from build123d import *

# Parameters (mm, degrees)
SKETCH1_W                    = 60
SKETCH1_H                    = 65
BASE_FLANGE1_DEPTH           = 0.5
CUT_EXTRUDE1_DEPTH           = 45.232341109
EDGE_FLANGE1_STRIP_W         = 2.2
EDGE_FLANGE1_STRIP_H         = 0.5
EDGE_FLANGE1_STRIP_CUT_DEPTH = 65
EDGE_FLANGE1_DEPTH           = 65
EXTRUDE_THIN1_START          = 38.85
EXTRUDE_THIN1_DEPTH          = 38.85
SKETCH87_W                   = 65
SKETCH87_H                   = 10
CUT_EXTRUDE2_DEPTH           = 30


# Sheet-metal steps are written as plain solids
with BuildPart() as part:
    # Sketch1 → Base-Flange1 (new body)
    with BuildSketch(Plane(origin=(0, 0, 0), x_dir=(1, 0, 0), z_dir=(0, 1, 0))):
        Rectangle(SKETCH1_W, SKETCH1_H)
    extrude(amount=-BASE_FLANGE1_DEPTH)

    # Sketch7 → Cut-Extrude1 (cut, through all)
    with BuildSketch(Plane.XZ.offset(0.5)):
        with BuildLine():
            Line((2, 32.5), (-30, 32.5))
            Line((-30, 32.5), (-30, -32.5))
            Line((-30, -32.5), (2, -32.5))
            ThreePointArc((2, -32.5), (-29.169489574, 0), (2, 32.5))
        make_face()
    extrude(amount=-CUT_EXTRUDE1_DEPTH, mode=Mode.SUBTRACT)

    # Edge-Flange1 strip (across the edge) → Edge-Flange1 strip cut (cut)
    with BuildSketch(Plane(origin=(30, -0.5, -32.5), x_dir=(-1, 0, 0), z_dir=(0, 0, 1))):
        with Locations((-0.5, -0.25)):
            Rectangle(EDGE_FLANGE1_STRIP_W, EDGE_FLANGE1_STRIP_H)
    extrude(amount=EDGE_FLANGE1_STRIP_CUT_DEPTH, mode=Mode.SUBTRACT)

    # Edge-Flange1 section (across the edge) → Edge-Flange1 (add)
    with BuildSketch(Plane(origin=(30, -0.5, -32.5), x_dir=(-1, 0, 0), z_dir=(0, 0, 1))):
        with BuildLine():
            Line((0, 0.1), (0, 38.85))
            Line((0, 38.85), (0.5, 38.85))
            Line((0.5, 38.85), (0.5, 0.1))
            ThreePointArc((0.5, 0.1), (0.529289322, 0.029289322), (0.6, 0))
            Line((0.6, 0), (0.6, -0.5))
            ThreePointArc((0.6, -0.5), (0.175735931, -0.324264069), (0, 0.1))
        make_face()
    extrude(amount=EDGE_FLANGE1_DEPTH)

    # Sketch84 → Extrude-Thin1 (add)
    with BuildSketch(Plane.XZ.offset(0.5).offset(EXTRUDE_THIN1_START)):
        with BuildLine():
            Line((29.5, 32.5), (2, 32.5))
            ThreePointArc((2, 32.5), (-29.169489574, 0), (2, -32.5))
            Line((2, -32.5), (29.5, -32.5))
            Line((29.5, -32.5), (29.5, -32))
            Line((29.5, -32), (2.010489053, -32))
            ThreePointArc((2.010489053, -32), (-28.669489574, 0), (2.010489053, 32))
            Line((2.010489053, 32), (29.5, 32))
            Line((29.5, 32), (29.5, 32.5))
        make_face()
    extrude(amount=-EXTRUDE_THIN1_DEPTH)

    # Sketch87 → Cut-Extrude2 (cut)
    with BuildSketch(Plane.ZY.offset(29.169489574)):
        with Locations((0, -21.5)):
            Rectangle(SKETCH87_W, SKETCH87_H)
    extrude(amount=-CUT_EXTRUDE2_DEPTH, mode=Mode.SUBTRACT)


solid = part.part
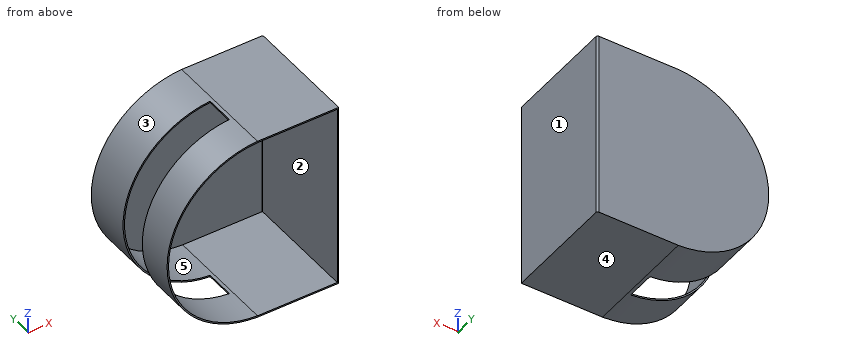
Work out the finished part from the listing and answer in its coordinate system (mm). Face numbers are marked on the shaded views. A direction names the side the tool comes from. Coordinates: 2 decimals unless noted, no trailing zeros. Write each loop counter-clockwise with the first axis right and the second up, starting at its lowest first coordinate (ties: lowest second). Pieces come first, ordered by that corner, then holes. Notation, with made-up numbers: M 26.5,31 L 79.5,31 A27 ccw 79.5,66 Z; hole C -26,-1.5 d3. An arc over 180 degrees is marked long. Use one line per item in the form item = value. Start each with the question number.
1. The part is cut by section D-D (y = -19). Give the vertices of the cut face in (x, z).
2. The part is cut by section B-B (y = -10.5). Give the vertices of the cut face in (x, z).
3. Each of these flat-tipped pins is pushed along its axis until it touches: P1, Ø8, axis at x = 17.5, z = 13, coming from the -Y side; P2, Ø1, axis at y = -30.5, z = -3.5, coming from the -X side; P3, Ø0.6, axis at y = -22, z = -32.5, coming from the -X side. Where does it stop, or does it pass through?
4. The part is cut by section C-C (x = -6.5). Give the vertices of the cut face in (y, z), plus the area to 3 significant figures.
5. Straight lines are drawn through the part: probe 1 along Z at (x, y) = (8, -19.5); probe 2 along Y at (x, z) = (-9.5, 8); probe 3 along Z at (x, y) = (-0.5, -9). For each, find the intervals that lie inside material, in ascending order. Write a range as from..to.
6. A tool of negligible diameter and unlimited length cuts with its end or side. For the marked faces 4 and 5, from which of +Z, -Z, +X, -X, +Y, -Y can it reach the whole face along a straight path? Write none if from no direction.
7. The part is cut by section A-A (z = -12). Give the vertices of the cut face in (x, y).
8. The mould has two halves that part along X. Classify the marked faces 1, 2 and 3: released by +X, released by -X, zero draft, split by the parting line, or undercut.
Evaluation:
q1.outline = M 0.83,-32.43 A32.53 ccw 2,-32.5 L 30,-32.5 L 30,32.5 L 2,32.5 A32.53 ccw 0.83,32.43 L 0.83,31.93 A32.03 cw 2.01,32 L 29.5,32 L 29.5,-32 L 2.01,-32 A32.03 cw 0.83,-31.93 Z
q2.outline = M 2,-32.5 L 30,-32.5 L 30,32.5 L 2,32.5 A32.53 ccw Z; hole M 2.01,-32 L 29.5,-32 L 29.5,32 L 2.01,32 A32.03 ccw Z
q3.P1 = -0.5
q3.P2 = -29.03
q3.P3 = 0.83
q4.outline = M -39.35,-31 L -26.5,-31 L -26.5,-30.47 L -39.35,-30.47 Z; M -39.35,30.47 L -26.5,30.47 L -26.5,31 L -39.35,31 Z; M -16.5,-31 L 0,-31 L 0,31 L -16.5,31 L -16.5,30.47 L -0.5,30.47 L -0.5,-30.47 L -16.5,-30.47 Z
q4.area = 61.3 mm^2
q5.probe_1 = -32.5..-32, 32..32.5
q5.probe_2 = -0.5..0
q5.probe_3 = -32.3..-31.8, 31.8..32.3
q6.face_4 = -Z, +X, -X, +Y, -Y
q6.face_5 = -Y
q7.outline = M -26.88,-39.35 L -26.34,-39.35 L -26.34,-26.5 L -26.88,-26.5 Z; M -26.88,-16.5 L -26.34,-16.5 L -26.34,-0.5 L 29.4,-0.5 A0.1 cw 29.5,-0.6 L 29.5,-39.35 L 30,-39.35 L 30,-0.6 A0.6 ccw 29.4,0 L -26.88,0 Z
q8.face_1 = released by +X
q8.face_2 = undercut
q8.face_3 = released by -X
